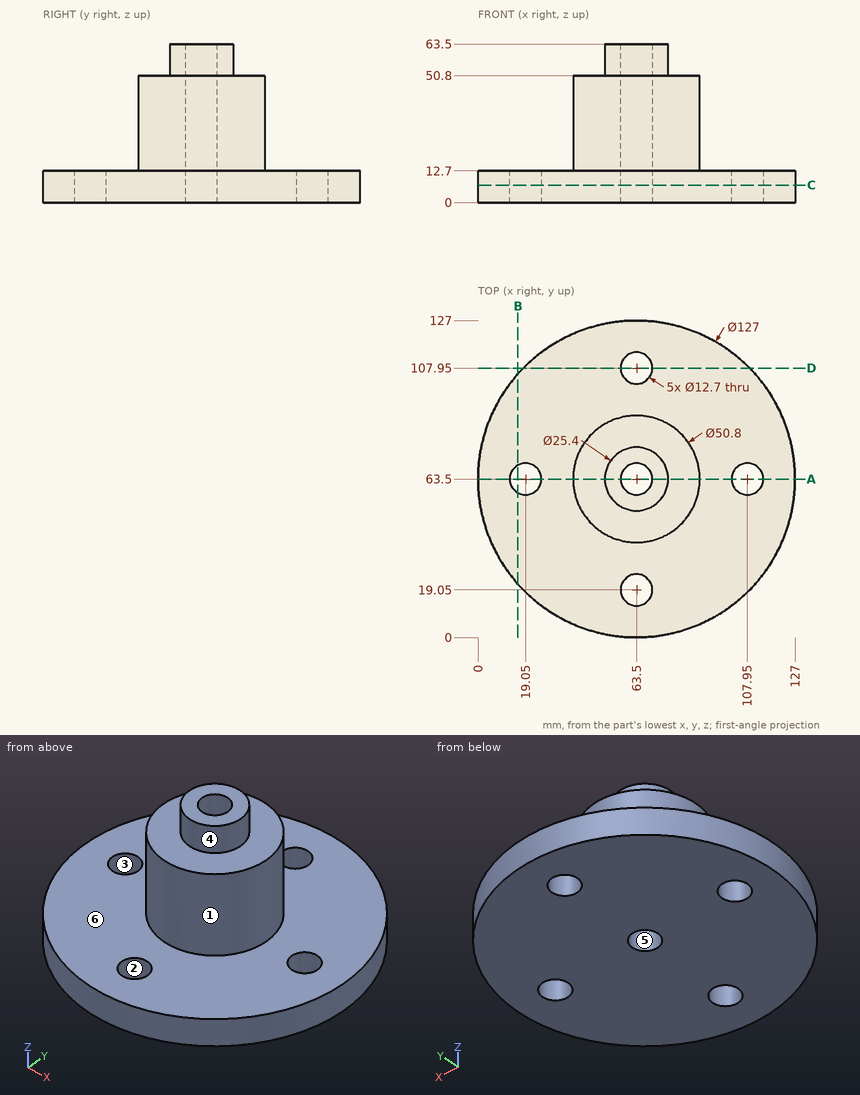
Drawing for the job (mm, zero at the part's lowest x, y, z). A direction names the side the tool comes from. Give positions to 0.01 mm unless a question says otherwise; leave off trailing zeros. Write each loop counter-clockwise with the first axis right and the second up, starting at its lowest first coordinate (ties: lowest second). Pieces come first, ordered by that corner, then holes. Notation, with made-up numbers: M 13,4.5 L 20,4.5 A26 ccw 20,20.5 Z; hole C -1.75,54.5 d6. An arc over 180 degrees is marked long. Return JSON: item names as keys, results as strings. Group by question number.
(1) Flat gauge pins, fed straight in: pin 1 Ø2 at (x, z) = (51.5, 19) entering from -Y; pin 2 Ø3 at (x, y) = (51, 40.5) entering from +Z; pin 3 Ø10 at (y, z) = (45.5, 52) entering from -X. Where does each tip first touch, or does it go through?
(2) 3-axis set-ups, long thin cutter, end or side, ignore diameter. For the marked faces 1 and 2: which of +Z, -Z, +X, -X, +Y, -Y reach the whole face in a straight line?
(3) Band-saw the part on D-D (y = 107.95). Give the cut face in (x, z), and give its area (3 significant figures).
(4) Drill centre lines: L1, parallel to Y at x = 63, z = 7; L2, parallel to Y at x = 63, z = 40; L3, parallel to Z at x = 114, y = 53. Where is each one in solid material? Low to high. Write a range as [from, to].
(5) Band-saw the part on C-C (z = 7). Give the cut face in (x, y), and give its area (3 significant figures).
(6) Band-saw the part on B-B (x = 16). Give the cut face in (y, z).
(7) Band-saw the part on A-A (y = 63.5). Give the cut face in (x, z), and give its area (3 significant figures).
(8) Mould opens along Y. For the marked faces 3, 4, 5 and 6 say: pulls with the +Y half, pulls with the -Y half, needs draft (parallel to the pull), parting line crosses it, or undercut.
Entries:
{
 "1": {"pin 1": "stops at y = 40.61", "pin 2": "stops at z = 50.8", "pin 3": "stops at x = 41.77"},
 "2": {"face 1": "+Z", "face 2": "+Z, -Z"},
 "3": {"outline": "M 18.15,0 L 57.15,0 L 57.15,12.7 L 18.15,12.7 Z; M 69.85,0 L 108.85,0 L 108.85,12.7 L 69.85,12.7 Z", "area": "991 mm^2"},
 "4": {"L1": "y = [0, 12.72], [25.38, 57.17], [69.83, 101.62], [114.28, 127]", "L2": "y = [38.1, 57.17], [69.83, 88.9]", "L3": "z = [0, 12.7]"},
 "5": {"outline": "C 63.5,63.5 d127; hole C 19.05,63.5 d12.7; hole C 63.5,19.05 d12.7; hole C 63.5,63.5 d12.7; hole C 63.5,107.95 d12.7; hole C 107.95,63.5 d12.7", "area": "12,000 mm^2"},
 "6": {"outline": "M 21.36,0 L 57.93,0 L 57.93,12.7 L 21.36,12.7 Z; M 69.07,0 L 105.64,0 L 105.64,12.7 L 69.07,12.7 Z"},
 "7": {"outline": "M 0,0 L 12.7,0 L 12.7,12.7 L 0,12.7 Z; M 25.4,0 L 57.15,0 L 57.15,63.5 L 50.8,63.5 L 50.8,50.8 L 38.1,50.8 L 38.1,12.7 L 25.4,12.7 Z; M 69.85,0 L 101.6,0 L 101.6,12.7 L 88.9,12.7 L 88.9,50.8 L 76.2,50.8 L 76.2,63.5 L 69.85,63.5 Z; M 114.3,0 L 127,0 L 127,12.7 L 114.3,12.7 Z", "area": "2,740 mm^2"},
 "8": {"face 3": "undercut", "face 4": "parting line crosses it", "face 5": "undercut", "face 6": "needs draft"}
}
